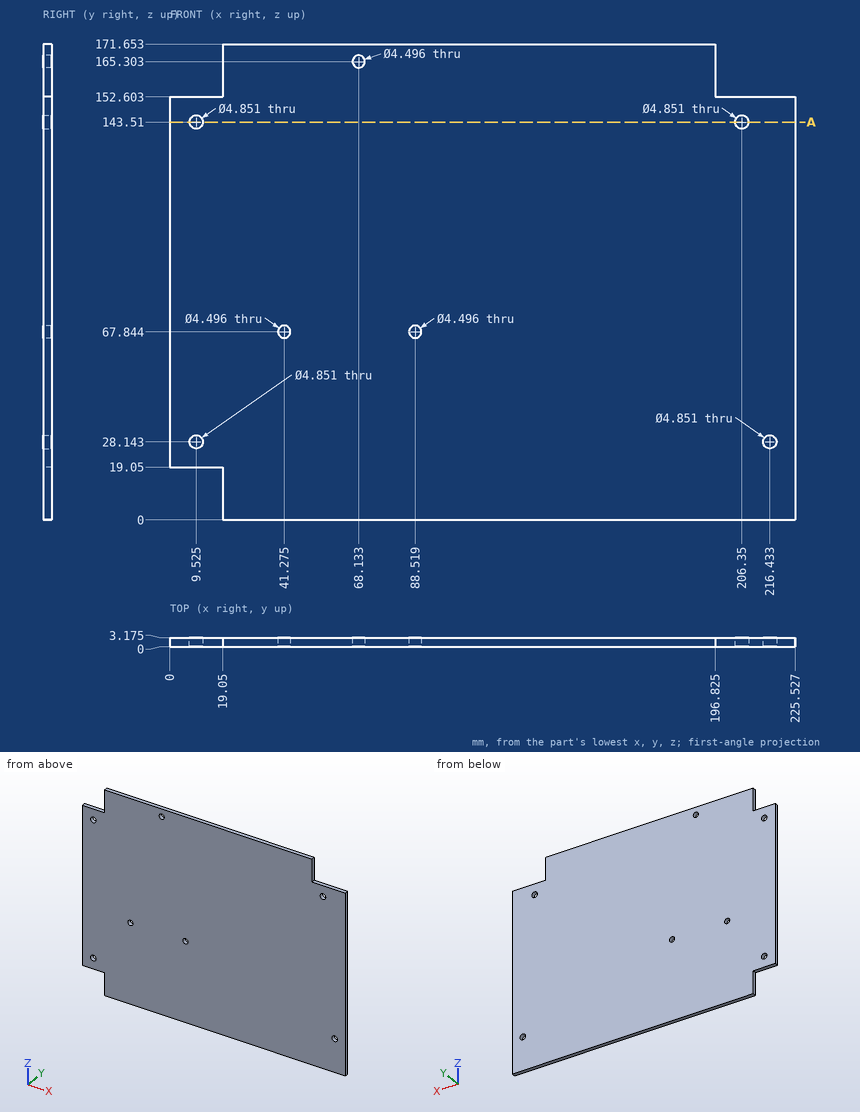
Here's the drawing with two shaded views (mm, measured from the low corner). I have some questions. Round coordinates to 2 decimals unless told otherwise and drop trailing zeros. Answer as a JSON object with one key per item and string values. Group by question number.
Q1. Imagine slicing it at A-A, the plane z = 143.51. Count the separate pieces of the cut face and the enclosed holes in it.
Q2. Please list where these lines run through material, in increasing order: L1, parallel to X at y = 2, z = 28 (1 decimal); L2, parallel to Z at x = 215, y = 1.8 (1 decimal); L3, parallel to Z at x = 212, y = 3.
Q3. Will these pins go through, and if not, where does the flat tip stop? pin 1 (3.5 mm diameter, centred on x = 88.52, z = 67.84, fed in from -Y); pin 2 (1.6 mm diameter, centred on y = 1.5, z = 10, fed in from -X); pin 3 (1 mm diameter, centred on x = 206, y = 2, fed in from +Z); pin 4 (1.6 mm diameter, centred on y = 1.5, z = 160, fed in from +X) (1 decimal).
Findings:
{
 "1": {"separate pieces": "3", "enclosed holes": "0"},
 "2": {"L1": "x = 0 to 7.1, 11.9 to 214, 218.9 to 225.5", "L2": "z = 0 to 26.2, 30.1 to 152.6", "L3": "z = 0 to 152.6"},
 "3": {"pin 1": "passes through", "pin 2": "stops at x = 19.05", "pin 3": "stops at z = 152.6", "pin 4": "stops at x = 196.8"}
}
